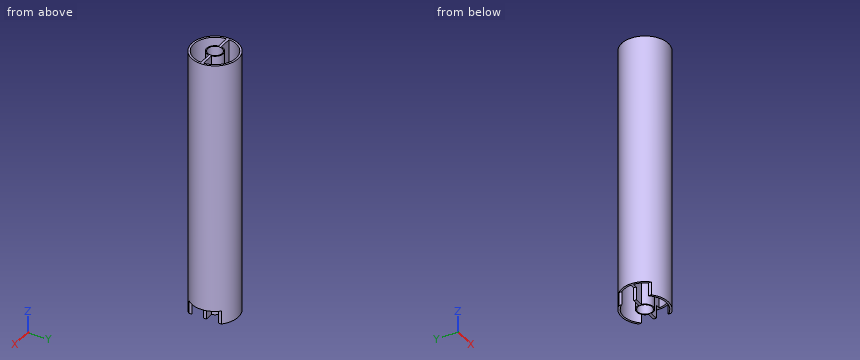
from build123d import *

# Parameters (mm, degrees)
SKETCH2_R                       = 17.5
SKETCH2_R_2                     = 5.5
SHELL_DEPTH                     = 200
SKETCH13_R                      = 16
SKETCH13_R_2                    = 6.25
SKETCH13_R_3                    = 4
INNERPARTITION_DEPTH            = 2.5
EASIERASSEMBLY_SHELLSTUDS_DEPTH = 10


with BuildPart() as part:
    # Sketch2 → Shell (new body)
    with BuildSketch(Plane.XY):
        Circle(SKETCH2_R)
        with BuildLine():
            Line((15.968719423, 1), (6.16948134, 1))
            ThreePointArc((6.16948134, 1), (0, 6.25), (-6.16948134, 1))
            Line((-6.16948134, 1), (-15.968719423, 1))
            ThreePointArc((-15.968719423, 1), (0, 16), (15.968719423, 1))
        make_face(mode=Mode.SUBTRACT)
        with BuildLine():
            ThreePointArc((-6.16948134, -1), (0, -6.25), (6.16948134, -1))
            Line((6.16948134, -1), (15.968719423, -1))
            ThreePointArc((15.968719423, -1), (0, -16), (-15.968719423, -1))
            Line((-15.968719423, -1), (-6.16948134, -1))
        make_face(mode=Mode.SUBTRACT)
        Circle(SKETCH2_R_2, mode=Mode.SUBTRACT)
    extrude(amount=SHELL_DEPTH)

    # Sketch13 → InnerPartition (add, symmetric)
    with BuildSketch(Plane.XY.offset(150)):
        Circle(SKETCH13_R)
        Circle(SKETCH13_R_2, mode=Mode.SUBTRACT)
        with Locations((0, 11.125)):
            Circle(SKETCH13_R_3, mode=Mode.SUBTRACT)
        with Locations((0, -11.125)):
            Circle(SKETCH13_R_3, mode=Mode.SUBTRACT)
    extrude(amount=INNERPARTITION_DEPTH, both=True)

    # Sketch2<18> → EasierAssembly_ShellStuds (cut)
    with BuildSketch(Plane.XY):
        with BuildLine():
            Line((12.5, 9.987492178), (12.5, 1))
            Line((12.5, 1), (15.968719423, 1))
            ThreePointArc((15.968719423, 1), (14.92684663, 5.76101117), (12.5, 9.987492178))
        make_face()
        with BuildLine():
            Line((-15.968719423, 1), (-12.5, 1))
            Line((-12.5, 1), (-12.5, 9.987492178))
            ThreePointArc((-12.5, 9.987492178), (-14.92684663, 5.76101117), (-15.968719423, 1))
        make_face()
        with BuildLine():
            ThreePointArc((-15.968719423, -1), (-14.92684663, -5.76101117), (-12.5, -9.987492178))
            Line((-12.5, -9.987492178), (-12.5, -1))
            Line((-12.5, -1), (-15.968719423, -1))
        make_face()
        with BuildLine():
            Line((12.5, -1), (12.5, -9.987492178))
            ThreePointArc((12.5, -9.987492178), (14.92684663, -5.76101117), (15.968719423, -1))
            Line((15.968719423, -1), (12.5, -1))
        make_face()
        with BuildLine():
            Line((12.5, 1), (12.5, -1))
            Line((12.5, -1), (15.968719423, -1))
            ThreePointArc((15.968719423, -1), (15.992177944, -0.500244559), (16, 0))
            ThreePointArc((16, 0), (15.992177944, 0.500244559), (15.968719423, 1))
            Line((15.968719423, 1), (12.5, 1))
        make_face()
        with BuildLine():
            Line((-15.968719423, -1), (-12.5, -1))
            Line((-12.5, -1), (-12.5, 1))
            Line((-12.5, 1), (-15.968719423, 1))
            ThreePointArc((-15.968719423, 1), (-16, 0), (-15.968719423, -1))
        make_face()
        with BuildLine():
            Line((-12.5, -12.247448714), (-12.5, -9.987492178))
            ThreePointArc((-12.5, -9.987492178), (-14.92684663, -5.76101117), (-15.968719423, -1))
            ThreePointArc((-15.968719423, -1), (-16, 0), (-15.968719423, 1))
            ThreePointArc((-15.968719423, 1), (-14.92684663, 5.76101117), (-12.5, 9.987492178))
            Line((-12.5, 9.987492178), (-12.5, 12.247448714))
            ThreePointArc((-12.5, 12.247448714), (-17.5, 0), (-12.5, -12.247448714))
        make_face()
        with BuildLine():
            ThreePointArc((15.968719423, -1), (14.92684663, -5.76101117), (12.5, -9.987492178))
            Line((12.5, -9.987492178), (12.5, -12.247448714))
            ThreePointArc((12.5, -12.247448714), (16.201851746, -6.614378278), (17.5, 0))
            ThreePointArc((17.5, 0), (16.201851746, 6.614378278), (12.5, 12.247448714))
            Line((12.5, 12.247448714), (12.5, 9.987492178))
            ThreePointArc((12.5, 9.987492178), (14.92684663, 5.76101117), (15.968719423, 1))
            ThreePointArc((15.968719423, 1), (15.992177944, 0.500244559), (16, 0))
            ThreePointArc((16, 0), (15.992177944, -0.500244559), (15.968719423, -1))
        make_face()
    extrude(amount=EASIERASSEMBLY_SHELLSTUDS_DEPTH, mode=Mode.SUBTRACT)


solid = part.part
Build history of the part. All positions in model axes, mm. Give positions to 0.01 mm unless a question says otherwise; leave off trailing zeros. Loops run counter-clockwise (first coordinate to the right, second up) from the corner with the lowest first, then second, coordinate; pieces in that order, holes last. Notation, with made-up numbers: (-17, 34.25) -> (-8, 34.25) arc R28 ccw to (-8, 67.25) -> close; hole circle Ø9 at (66.5, 19.25). An arc over 180 degrees is marked (long way). Answer in a Markdown table with one row per item.
Item 1: Slice it at A-A on z = 76. Write the cut outline in (x, y).
Findings below:
| item | result |
|---|---|
| outline | circle Ø35 at (0, 0); hole (-15.97, -1) arc R16 ccw to (15.97, -1) -> (6.17, -1) arc R6.25 cw to (-6.17, -1) -> close; hole (-15.97, 1) -> (-6.17, 1) arc R6.25 cw to (6.17, 1) -> (15.97, 1) arc R16 ccw to start; hole circle Ø11 at (0, 0) |
Item 2: Flat gauge pins, fed straight in: P1, Ø11, axis at x = 13, z = 180.5, coming from the -Y side; P2, Ø1, axis at x = -6.5, z = 31, coming from the -Y side; P3, Ø9, axis at x = 0, y = 11.125, coming from the -Z side. Where does each tip first touch, or does it go through?
Findings below:
| item | result |
|---|---|
| P1 | stops at y = -15.81 |
| P2 | stops at y = -16.44 |
| P3 | stops at z = 147.5 |
Item 3: Slice it at D-D on x = 10.5. Write the cut outline in (y, z), plus the area to 3 significant figures.
Findings below:
| item | result |
|---|---|
| outline | (-14, 0) -> (-12.07, 0) -> (-12.07, 147.5) -> (-1, 147.5) -> (-1, 0) -> (1, 0) -> (1, 147.5) -> (12.07, 147.5) -> (12.07, 0) -> (14, 0) -> (14, 200) -> (12.07, 200) -> (12.07, 152.5) -> (1, 152.5) -> (1, 200) -> (-1, 200) -> (-1, 152.5) -> (-12.07, 152.5) -> (-12.07, 200) -> (-14, 200) -> close |
| area | 1,280 mm² |
Item 4: Slice it at B-B on x = 0. Give the number of separate pieces and of enclosed holes in the cut face, plus the area to 4 significant figures.
Findings below:
| item | result |
|---|---|
| separate pieces | 4 |
| enclosed holes | 0 |
| area | 917.5 mm² |
Item 5: Slice it at C-C on y = 3. Write the cut outline in (x, z).
Findings below:
| item | result |
|---|---|
| outline | (-17.24, 10) -> (-15.72, 10) -> (-15.72, 147.5) -> (-5.48, 147.5) -> (-5.48, 0) -> (-4.61, 0) -> (-4.61, 200) -> (-5.48, 200) -> (-5.48, 152.5) -> (-15.72, 152.5) -> (-15.72, 200) -> (-17.24, 200) -> close; (4.61, 0) -> (5.48, 0) -> (5.48, 147.5) -> (15.72, 147.5) -> (15.72, 10) -> (17.24, 10) -> (17.24, 200) -> (15.72, 200) -> (15.72, 152.5) -> (5.48, 152.5) -> (5.48, 200) -> (4.61, 200) -> close |
Item 6: Probe line 1 along Y through (x, z) = (0, 94); line 2 along Y through (x, z) = (0, 149.3) (3 decimals); line 3 along Y through (x, z) = (-7, 160.5). List the from-to ranges inside material, lowest first. Write a range as [from, to].
Findings below:
| item | result |
|---|---|
| line 1 | y = [-17.5, -16], [-6.25, -5.5], [5.5, 6.25], [16, 17.5] |
| line 2 | y = [-17.5, -15.125], [-7.125, -5.5], [5.5, 7.125], [15.125, 17.5] |
| line 3 | y = [-16.04, -14.39], [-1, 1], [14.39, 16.04] |
